Input: part model. Units: mm. Frame: model coordinates. Round coordinates to 2 decimals unless told otherwise and drop trailing zeros. Loops run counter-clockwise (first coordinate to the right, second up) from the corner with the lowest first, then second, coordinate; pieces in that order, holes last. Notation, with made-up numbers: (71, 60.5) - (121, 60.5) arc R11 cw to (121, 71.5) - close; hole circle Ø8 at (23.25, 44.5). An arc over 180 degrees is marked (long way). Write each question's results on one line, items separated by ' | '.
from build123d import *

# Parameters (mm, degrees)
F0_W     = 38.277834
F0_H     = 285.75
F1_DEPTH = 1371.6
F2_SIZE  = 38.1
F3_W     = 1333.5
F3_H     = 19.05
F4_DEPTH = 19.05


with BuildPart() as f1:
    # F0 (on Front) → F1 (new body)
    with BuildSketch(Plane.XZ):
        Rectangle(F0_W, F0_H)
    extrude(amount=F1_DEPTH)

    # F2
    f2_edges = [f1.edges().sort_by_distance(p)[0] for p in [
        (19.138917, -1371.6, 0),
        (19.138917, 0, 0),
    ]]
    chamfer(f2_edges, length=F2_SIZE)

    # F3 (on face) → F4 (cut)
    with BuildSketch(Plane.YZ.offset(19.138917)):
        with Locations((-685.8, 133.35)):
            Rectangle(F3_W, F3_H)
    extrude(amount=-F4_DEPTH, mode=Mode.SUBTRACT)


solid = f1.part
1. Line query: line 1 (Z direction, x = 6, y = -355) (3 decimals); line 2 (X direction, y = -82, z = 127); line 3 (Y direction, x = -16, z = -8.5). Output: solid intervals per line, ascending. Write a range as [from, to].
Answer:
line 1: [-142.875, 123.825] | line 2: [-19.14, 0.09] | line 3: [-1368.64, -2.96]
2. Section query C-C, the plane x = 8. Output: boundary loops of the cut face in (y, z) (3 decimals).
Answer:
outline: (-1344.639, -142.875) - (-26.961, -142.875) - (-26.961, 123.825) - (-1344.639, 123.825) - close
3. Contact query for flat-ended pins moving along their axis: pin 1 (12 mm diameter, centred on x = -3, z = -85, fed in from -Y); pin 2 (15 mm diameter, centred on x = 13, y = -866, fed in from +Z) (3 decimals); pin 3 (5.5 mm diameter, centred on y = -569.5, z = 131.5, fed in from +X). Output: stop coordinate, or through.
Answer:
pin 1: y = -1361.64 | pin 2: z = 123.825 | pin 3: x = 0.09
4. Section query B-B, the plane y = -1222. Output: boundary loops of the cut face in (x, z) (3 decimals).
Answer:
outline: (-19.139, -142.875) - (19.139, -142.875) - (19.139, 123.825) - (0.089, 123.825) - (0.089, 142.875) - (-19.139, 142.875) - close
5. Section query A-A, the plane z = 36. Output: boundary loops of the cut face in (x, y).
Answer:
outline: (-19.14, -1371.6) - (-18.96, -1371.6) - (19.14, -1333.5) - (19.14, -38.1) - (-18.96, 0) - (-19.14, 0) - close
